```python
from build123d import *

# Parameters (mm, degrees)
BOSS_EXTRUDE1_DEPTH             = 45.212
SKETCH1_3_W                     = 90.17
SKETCH1_3_H                     = 69.85
SKETCH1_3_R                     = 1.5494
BOSS_EXTRUDE2_DEPTH             = 5.08
SKETCH1_4_R                     = 1.5494
BOSS_EXTRUDE3_DEPTH             = 5.08
FILLET1_R                       = 2.54
F_2_56_TAPPED_HOLE1_D           = 1.778
F_2_56_TAPPED_HOLE1_DEPTH       = 5.588
F_2_56_TAPPED_HOLE1_CSINK_D     = 3.4544
F_2_56_TAPPED_HOLE1_CSINK_ANGLE = 90
F_2_56_TAPPED_HOLE1_TIP         = 0.53416509
FILLET3_R                       = 2.54
FILLET4_R                       = 2.54


with BuildPart() as part:
    # Sketch1 → Boss-Extrude1 (new body)
    with BuildSketch(Plane(origin=(0, 0, 0), x_dir=(1, 0, 0), z_dir=(0, 1, 0))):
        Polygon((-62.865, -52.705), (201.232093857, -52.705), (-62.865, 132.217775938), align=None)
        Polygon((185.120392261, -47.625), (-57.785, 122.459186733), (-57.785, -47.625), align=None, mode=Mode.SUBTRACT)
    extrude(amount=BOSS_EXTRUDE1_DEPTH)

    # Sketch1_3 → Boss-Extrude2 (add)
    # profile 1 of 7: a face of its own
    with BuildSketch(Plane(origin=(0, 0, 0), x_dir=(1, 0, 0), z_dir=(0, 1, 0))):
        Polygon((-62.865, -52.705), (201.232093857, -52.705), (-62.865, 132.217775938), align=None)
        Polygon((185.120392261, -47.625), (-57.785, 122.459186733), (-57.785, -47.625), align=None, mode=Mode.SUBTRACT)
    # profile 2 of 7: a face of its own
    with BuildSketch(Plane(origin=(0, 0, 0), x_dir=(1, 0, 0), z_dir=(0, 1, 0))):
        Polygon((-57.785, -47.625), (185.120392261, -47.625), (-57.785, 122.459186733), align=None)
        Rectangle(SKETCH1_3_W, SKETCH1_3_H, mode=Mode.SUBTRACT)
    # profile 3 of 7: a face of its own
    with BuildSketch(Plane(origin=(0, 0, 0), x_dir=(1, 0, 0), z_dir=(0, 1, 0))):
        Rectangle(SKETCH1_3_W, SKETCH1_3_H)
        with Locations((-41.6052, -32.4104)):
            Circle(SKETCH1_3_R, mode=Mode.SUBTRACT)
        with Locations((41.7068, -32.3596)):
            Circle(SKETCH1_3_R, mode=Mode.SUBTRACT)
        with Locations((41.8846, 32.639)):
            Circle(SKETCH1_3_R, mode=Mode.SUBTRACT)
        with Locations((-41.656, 32.6136)):
            Circle(SKETCH1_3_R, mode=Mode.SUBTRACT)
    # profile 4 of 7: a face of its own
    with BuildSketch(Plane(origin=(0, 0, 0), x_dir=(1, 0, 0), z_dir=(0, 1, 0))):
        with Locations((-41.6052, -32.4104)):
            Circle(SKETCH1_3_R)
    # profile 5 of 7: a face of its own
    with BuildSketch(Plane(origin=(0, 0, 0), x_dir=(1, 0, 0), z_dir=(0, 1, 0))):
        with Locations((41.8846, 32.639)):
            Circle(SKETCH1_3_R)
    # profile 6 of 7: a face of its own
    with BuildSketch(Plane(origin=(0, 0, 0), x_dir=(1, 0, 0), z_dir=(0, 1, 0))):
        with Locations((41.7068, -32.3596)):
            Circle(SKETCH1_3_R)
    # profile 7 of 7: a face of its own
    with BuildSketch(Plane(origin=(0, 0, 0), x_dir=(1, 0, 0), z_dir=(0, 1, 0))):
        with Locations((-41.656, 32.6136)):
            Circle(SKETCH1_3_R)
    extrude(amount=-BOSS_EXTRUDE2_DEPTH)

    # Sketch1_4 → Boss-Extrude3 (add)
    with BuildSketch(Plane(origin=(0, 0, 0), x_dir=(1, 0, 0), z_dir=(0, 1, 0))):
        with Locations(Location((41.8846, 32.639, 0), (0, 0, 270))):
            Circle(SKETCH1_4_R)
        with Locations(Location((41.7068, -32.3596, 0), (0, 0, 270))):
            Circle(SKETCH1_4_R)
        with Locations(Location((-41.6052, -32.4104, 0), (0, 0, 270))):
            Circle(SKETCH1_4_R)
        with Locations(Location((-41.656, 32.6136, 0), (0, 0, 270))):
            Circle(SKETCH1_4_R)
    extrude(amount=BOSS_EXTRUDE3_DEPTH)

    # Fillet1
    fillet1_edges = [part.edges().sort_by_distance(p)[0] for p in [
        (-62.865, 20.066, 52.705),
        (-62.865, 20.066, -132.217775938),
        (201.232093857, 20.066, 52.705),
        (-57.785, 22.606, -122.459186733),
        (-57.785, 22.606, 47.625),
        (185.120392261, 22.606, 47.625),
    ]]
    fillet(fillet1_edges, radius=FILLET1_R)

    # 2-56 Tapped Hole1
    with Locations(Plane(origin=(0, 5.08, 0), x_dir=(1, 0, 0), z_dir=(0, 1, 0))):
        with Locations((41.8846, 32.639), (-41.656, 32.6136), (41.7068, -32.3596), (-41.656, -32.3596)):
            CounterSinkHole(F_2_56_TAPPED_HOLE1_D / 2, F_2_56_TAPPED_HOLE1_CSINK_D / 2, depth=F_2_56_TAPPED_HOLE1_DEPTH, counter_sink_angle=F_2_56_TAPPED_HOLE1_CSINK_ANGLE)
            with Locations((0, 0, -(F_2_56_TAPPED_HOLE1_DEPTH + F_2_56_TAPPED_HOLE1_TIP / 2))):  # 118° drill point
                Cone(0, F_2_56_TAPPED_HOLE1_D / 2, F_2_56_TAPPED_HOLE1_TIP, mode=Mode.SUBTRACT)

    # Fillet3
    fillet3_edges = [part.edges().sort_by_distance(p)[0] for p in [
        (-62.865, -5.08, -38.586740668),
        (66.425621529, -5.08, 52.705),
        (67.882505678, -5.08, -40.66738686),
        (-62.121051224, -5.08, 51.961051224),
        (195.598684114, -5.08, 50.928792731),
        (-61.497841478, -5.08, -129.591488852),
    ]]
    fillet(fillet3_edges, radius=FILLET3_R)

    # Fillet4
    fillet4_edges = [part.edges().sort_by_distance(p)[0] for p in [
        (-57.785, 0, -36.247446065),
        (60.909770731, 0, 47.625),
        (62.36665488, 0, -38.328092258),
        (-56.417841478, 0, -119.832899647),
        (179.486982518, 0, 45.848792731),
        (-57.041051224, 0, 46.881051224),
    ]]
    fillet(fillet4_edges, radius=FILLET4_R)


solid = part.part
```
The model under review builds one solid part; all positions refer to its coordinate system, in mm. A direction names the side the tool comes from. Round coordinates to 2 decimals unless told otherwise and drop trailing zeros. Write each loop counter-clockwise with the first axis right and the second up, starting at its lowest first coordinate (ties: lowest second). Pieces come first, ordered by that corner, then holes. Notation, with made-up numbers: (75.25, 74.5) - (109.25, 74.5) arc R20 ccw to (109.25, 110.5) - close; hole circle Ø5 at (-31, 0.5). An arc over 180 degrees is marked (long way). Answer as CSV lines item,"result". Start each with the question number.
(1) We need section A-A on y = 39.5. State the section outline as (x, z) points (3 decimals), plus the area to 3 significant figures.
(2) For faces 1 (the flat face through (59, 24, 47.625)), 2 (the flat face through (-62.865, 22, -40)), list the 3-axis set-ups (+Z, -Z, +X, -X, +Y, -Y) from which the entire face can be reached by the end or side of a thin tool; tool diameter is ignored.
(3) Draft analysis for pull direction Z (two halves, no side actions). For faces 3 (the flat face through (69.657, 21.67, -39.425)), 4 (the cylindrical face through (60.325, 0.764, -38.873)), 5 (the flat face through (8, -5.08, 0)), state which applies: pulls with the +Z half, pulls with the -Z half, needs draft (parallel to the pull), parting line crosses it, or undercut.
(4) For pin 1 Ø3 at (y, z) = (32, -18.5) entering from +X; pin 2 Ø1 at (x, y) = (57.5, 21.5) entering from -Z; pin 3 Ø6 at (y, z) = (39.5, -70) entering from +X, all flat-tipped, find the tip position at first contact; note any pin that passes through.
(5) To check wall thickness, follow line 1 (Y direction, x = -2, z = -35); line 2 (X direction, y = 17, z = -38) (3 decimals); line 3 (Z direction, x = 183.5, y = 37) (3 decimals). State the ranges of each line that lie inside material, in increasing order.
Worked answers:
1,outline,"(-62.865, -127.338) arc R2.54 ccw to (-58.868, -129.419) - (194.633, 48.084) arc R2.54 ccw to (193.176, 52.705) - (-60.325, 52.705) arc R2.54 ccw to (-62.865, 50.165) - close; hole (-57.785, -117.58) arc R2.54 ccw to (-53.788, -119.661) - (178.521, 43.004) arc R2.54 ccw to (177.065, 47.625) - (-55.245, 47.625) arc R2.54 ccw to (-57.785, 45.085) - close"
1,area,"3,760 mm²"
2,face 1,"+Y"
2,face 2,"+Z, -Z, -X, +Y, -Y"
3,face 3,"pulls with the -Z half"
3,face 4,"undercut"
3,face 5,"needs draft"
4,pin 1,"x = 101.68"
4,pin 2,"z = -48.29"
4,pin 3,"x = 30.28"
5,line 1,"-5.08 to 0"
5,line 2,"-62.865 to -57.785, 62.835 to 71.692"
5,line 3,"40.289 to 52.705"
